```python
from build123d import *

# Parameters (mm, degrees)
F1_DEPTH    = 2.54
F2_T4_DEPTH = 40.6971516331
F3_T4_DEPTH = 48.3394519199
F4_T4_DEPTH = 63.1242461628


# Not quite as in the source:
# - a fillet or chamfer that OpenCascade refuses, or shapes differently, is made with other operations: its cross-section is extruded or revolved along the edge and cut away or added


with BuildPart() as f1:
    # F0 (on Right) → F1 (new body)
    with BuildSketch(Plane.YZ):
        Polygon((-0.3011617849, 0), (-4.707176704, 0), (-4.707176704, -3.2687797211), (-4.707176704, -9.6434028819), (-4.707176704, -62.8868843283), (0, -62.8868843283), (0, -10.7670552097), align=None)
        with BuildLine():
            Line((-4.707176704, -9.6434028819), (-4.707176704, -3.2687797211))
            Line((-4.707176704, -3.2687797211), (-8.1328889355, -3.2687797211))
            Line((-8.1328889355, -3.2687797211), (-16.7150776833, 8.5039641708))
            ThreePointArc((-16.7150776833, 8.5039641708), (-18.448774527, -6.0153747507), (-18.2778015733, -20.6368546933))
            Line((-18.2778015733, -20.6368546933), (-8.4392093122, -9.6434028819))
            Line((-8.4392093122, -9.6434028819), (-4.707176704, -9.6434028819))
        make_face()
        Polygon((0, 0), (-0.3011617849, 0), (0, -10.7670552097), (21.1573056877, -4.0066023357), align=None)
    extrude(amount=F1_DEPTH)

    # F2: chamfer of 5.08 on 1 edges, made by hand


with BuildPart() as f2_tool2:
    # F2_s3 → F2_t4 (new body)
    with BuildSketch(Plane(origin=(0, 6.4295894432, -8.8198840726), x_dir=(1, 0, 0), z_dir=(0, -0.5890778812, 0.8080762649))):
        Polygon((-2.54, -8.497560346), (2.54, -13.577560346), (2.54, -8.497560346), align=None)
    extrude(amount=F2_T4_DEPTH)

    split(bisect_by=Plane.XY.offset(-3.2687797211), keep=Keep.TOP)


with BuildPart() as f1_1:
    add(f1.part)

    # F2_t1: cut F2_tool2
    add(f2_tool2.part, mode=Mode.SUBTRACT)

    # F3: chamfer of 5.08 on 1 edges, made by hand


with BuildPart() as f3_tool2:
    # F3_s3 → F3_t4 (new body)
    with BuildSketch(Plane(origin=(0, -15.5659961488, -4.9738461482), x_dir=(1, 0, 0), z_dir=(0, 0.9525532472, 0.3043719948))):
        Polygon((2.54, 5.1761934028), (-2.54, 10.2561934028), (2.54, 10.2561934028), align=None)
    extrude(amount=F3_T4_DEPTH)

    split(bisect_by=Plane.XZ, keep=Keep.BOTTOM)


with BuildPart() as f1_2:
    add(f1_1.part)

    # F3_t1: cut F3_tool2
    add(f3_tool2.part, mode=Mode.SUBTRACT)

    # F4: chamfer of 5.08 on 1 edges, made by hand


with BuildPart() as f4_tool2:
    # F4_s3 → F4_t4 (new body)
    with BuildSketch(Plane(origin=(0, 23.513886354, -4.4528728458), x_dir=(1, 0, 0), z_dir=(0, -0.9825374139, 0.1860651236))):
        Polygon((2.54, -5.08), (-2.54, 0), (2.54, 0), align=None)
    extrude(amount=F4_T4_DEPTH)

    split(bisect_by=Plane(origin=(-5.518780173, -4.4595952689, -3.2509913312), x_dir=(-0.6285178248, 0.7777951812, 0), z_dir=(0.7071067812, 0.5713962066, 0.4165409645)), keep=Keep.TOP)


with BuildPart() as f1_3:
    add(f1_2.part)

    # F4_t1: cut F4_tool2
    add(f4_tool2.part, mode=Mode.SUBTRACT)


solid = f1_3.part
```
CAD build for the part. Positions are in the model's coordinates, mm. A direction names the side the tool comes from. Round coordinates to 2 decimals unless told otherwise and drop trailing zeros. Order: outer loops, then holes, each group sorted by start corner. A loop starts at its lowest first (then second) coordinate and runs counter-clockwise, first axis right, second up. Notation, with made-up numbers: (76.25, -17) - (114.25, -17) arc R23 cw to (114.25, 20) - close; hole circle Ø6 at (76.25, 46.25). An arc over 180 degrees is marked (long way). Answer in a Markdown table with one row per item. Add a question column.
(1) Band-saw the part on C-C on z = -52.5. List the corners of the cut face in (x, y).
(2) Band-saw the part on B-B on x = 0.45. List the corners of the cut face in (y, z).
(3) Probe L1, parallel to Y at x = 0.4, z = -32; L2, parallel to Y at x = 1, z = -10; L3, parallel to Z at x = 0.8, y = -11.75. List the from-to ranges inside material, lowest first. Write a range as [from, to].
(4) 3-axis set-ups, long thin cutter, end or side, ignore diameter. For faces 1 (the face through (0.4, -4.707, -2.8)), 2 (the face through (1, -4.707, -36)), 3 (the face through (0.72, 3.92, -6.09)), 4 (the face through (1, -9, -3.269)), 5 (the face through (2.54, -4, -26)): which of +Z, -Z, +X, -X, +Y, -Y reach the whole face in a straight line?
(5) Mould opens along Y. For faces 6 (the face through (1.29, 0.54, -4)), 7 (the face through (1, -7, -9.643)), 8 (the face through (0, -4, -21)) say: +Y half, -Y half, draft (parallel to the pull), parting line (faces both ways), or undercut.
(6) Drop flat-ended pins along their axis: pin 1 Ø1.5 at (x, y) = (1, -12) entering from -Z; pin 2 Ø1.3 at (x, z) = (0.5, -34) entering from +Y; pin 3 Ø1.3 at (x, z) = (2, -23) entering from -Y. Give the stop position or say it passes through.
(7) Band-saw the part on A-A on z = -12.5. List the corners of the cut face in (x, y).
(8) Band-saw the part on D-D on y = -13. List the corners of the cut face in (x, z).
Data:
| question | item | result |
|---|---|---|
| 1 | outline | (0, -4.71) - (2.54, -4.71) - (2.54, 0) - (0, 0) - close |
| 2 | outline | (-18.28, -20.64) - (-8.44, -9.64) - (-4.71, -9.64) - (-4.71, -62.89) - (0, -62.89) - (0, -7.63) - (9.01, -4.75) - (-4.71, -2.15) - (-4.71, -3.27) - (-11.83, -3.27) - (-17.4, 4.37) arc R112.1 ccw to start |
| 3 | L1 | y = [-4.71, 0] |
| 3 | L2 | y = [-18.59, -8.76], [-4.71, 0] |
| 3 | L3 | z = [-13.34, -3.27] |
| 4 | face 1 | +Z, +X, -X |
| 4 | face 2 | -Z, +X, -X |
| 4 | face 3 | -Z, +X, +Y |
| 4 | face 4 | +Z, +X |
| 4 | face 5 | +Z, -Z, +X, +Y, -Y |
| 5 | face 6 | +Y half |
| 5 | face 7 | undercut |
| 5 | face 8 | draft |
| 6 | pin 1 | stops at z = -14.46 |
| 6 | pin 2 | stops at y = 0 |
| 6 | pin 3 | stops at y = -4.71 |
| 7 | outline | (0, -18.61) - (2.54, -18.61) - (2.54, -11) - (0, -11) - close; (0, -4.71) - (2.54, -4.71) - (2.54, 0) - (0, 0) - close |
| 8 | outline | (0, -14.74) - (2.54, -14.74) - (2.54, -3.27) - (1.39, -3.27) - (0, -0.9) - close |
